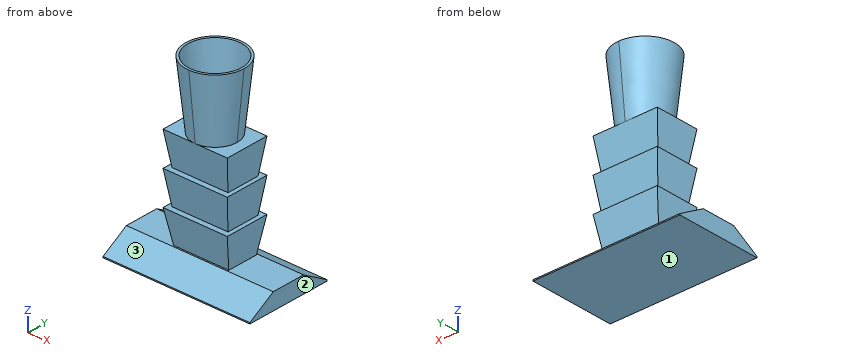
```python
from build123d import *

# Parameters (mm, degrees)
F0_W      = 60.96
F0_H      = 35.56
F1_DEPTH  = 6.858
F2_SIZE2  = 6.3754
F2_SIZE   = 10.795
F3_W      = 22.86
F3_H      = 12.7
F5_W      = 26.67
F5_H      = 18.288
F8_W      = 23.241
F8_H      = 13.843
F9_W      = 26.67
F9_H      = 18.288
F12_W     = 23.241
F12_H     = 13.843
F13_W     = 26.67
F13_H     = 18.288
F17_R     = 12.065
F19_R     = 11.0998
F20_DEPTH = 27.432
F20_TAPER = 6


with BuildPart() as f1:
    # F0 (on Top) → F1 (new body)
    with BuildSketch(Plane.XY):
        Rectangle(F0_W, F0_H)
    extrude(amount=F1_DEPTH)

    # F2
    f2_edges = [f1.edges().sort_by_distance(p)[0] for p in [
        (0, 17.78, 6.858),
        (0, -17.78, 6.858),
    ]]
    f2_side = f1.faces().sort_by_distance((0, 0, 6.858))[0]
    chamfer(f2_edges, length=F2_SIZE, length2=F2_SIZE2, reference=f2_side)

    # F3 (on face) → F6 section 0
    with BuildSketch(Plane.XY.offset(6.858)):
        Rectangle(F3_W, F3_H)
    # F5 (on offset) → F6 section 1
    with BuildSketch(Plane.XY.offset(20.828)):
        Rectangle(F5_W, F5_H)
    loft()

    # F8 (on face) → F10 section 0
    with BuildSketch(Plane.XY.offset(20.828)):
        Rectangle(F8_W, F8_H)
    # F9 (on offset) → F10 section 1
    with BuildSketch(Plane.XY.offset(34.798)):
        Rectangle(F9_W, F9_H)
    loft()

    # F12 (on face) → F14 section 0
    with BuildSketch(Plane.XY.offset(34.798)):
        Rectangle(F12_W, F12_H)
    # F13 (on offset) → F14 section 1
    with BuildSketch(Plane.XY.offset(48.768)):
        Rectangle(F13_W, F13_H)
    loft()

    # F15 (on face) → F18 section 0
    with BuildSketch(Plane.XY.offset(48.768)):
        with BuildLine():
            ThreePointArc((0, 9.144), (-9.144, 0), (0, -9.144))
            ThreePointArc((0, -9.144), (6.4657844072, -6.4657844072), (9.144, 0))
            ThreePointArc((9.144, 0), (6.4657844072, 6.4657844072), (0, 9.144))
        make_face()
    # F17 (on offset) → F18 section 1
    with BuildSketch(Plane.XY.offset(76.2)):
        Circle(F17_R)
    loft()

    # F19 (on face) → F20 (cut, through all)
    with BuildSketch(Plane.XY.offset(76.2)):
        Circle(F19_R)
    extrude(amount=-F20_DEPTH, taper=F20_TAPER, mode=Mode.SUBTRACT)


solid = f1.part
```
Input: part model. Units: mm. Frame: model coordinates. Face numbers are marked on the shaded views. Give positions to 0.01 mm unless a question says otherwise; leave off trailing zeros. Order: outer loops, then holes, each group sorted by start corner. A loop starts at its lowest first (then second) coordinate and runs counter-clockwise, first axis right, second up.
1. Section A-A on x = -23.5. Return the cut outline in (y, z) (3 decimals), and give its area (3 significant figures).
Derived:
outline: (-17.78, 0) - (17.78, 0) - (17.78, 0.483) - (6.985, 6.858) - (-6.985, 6.858) - (-17.78, 0.483) - close
area: 175 mm2
2. Mould query, pull axis Z, two halves, no side actions, for the marked faces 1, 2 and 3. Classes: released by +Z, released by -Z, zero draft, split by the parting line, or undercut.
Derived:
face 1: released by -Z
face 2: zero draft
face 3: undercut
3. Section B-B on z = 64. Return the cut outline in (x, y).
Derived:
outline: circle Ø21.53 at (0, 0); hole circle Ø19.64 at (0, 0)
4. Section C-C on y = 13.5. Return the cut outline in (x, z), and give its area (3 significant figures).
Derived:
outline: (-30.48, 0) - (30.48, 0) - (30.48, 3.01) - (-30.48, 3.01) - close
area: 184 mm2
5. Pin query (flat end, axial travel): pin 1 (4 mm diameter, centred on x = 1.5, z = 22, fed in from +Y); pin 2 (4 mm diameter, centred on x = 15.5, y = 4, fed in from -Z); pin 3 (1.5 mm diameter, centred on x = 1.5, z = 8, fed in from +Y); pin 4 (6 mm diameter, centred on x = -16.5, y = -9, fed in from +Z). Return the tip coordinate at first contact, or that it passes through.
Derived:
pin 1: stops at y = 9.14
pin 2: stops at z = 0
pin 3: stops at y = 6.73
pin 4: stops at z = 6.86
6. Section D-D on z = 51. Return the cut outline in (x, y).
Derived:
outline: circle Ø18.76 at (0, 0); hole circle Ø16.9 at (0, 0)
7. Material intervals for L1, parallel to X at y = 8.5, z = 59; L2, parallel to X at y = -7, z = 72.5; L3, parallel to Z at x = 6, y = -4, sorted ascending.
Derived:
L1: x = -5.7 to -3.75, 3.75 to 5.7
L2: x = -9.34 to -8.11, 8.11 to 9.34
L3: z = 0 to 48.77
